```python
from build123d import *

# Parameters (mm, degrees)
M6X0P35_MALE_THREAD_MAJOR_ENVELOPE_START = 0.8
SKETCH1_R                                = 3
SKETCH1_R_2                              = 2.2
M6X0P35_MALE_THREAD_MAJOR_ENVELOPE_DEPTH = 1.4
BALL_RETENTION_CAP_FLANGE_START          = 2.2
SKETCH2_R                                = 3.5
SKETCH2_R_2                              = 2.2
BALL_RETENTION_CAP_FLANGE_DEPTH          = 0.5
SKETCH3_W                                = 0.45
SKETCH3_H                                = 0.6
OPPOSED_PIN_TOOL_NOTCHES_DEPTH           = 0.5


# Read off the part's stored shape, not the designer's step: Upper_Spherical_Bearing_Seat_D5p05
with BuildPart() as part:
    # Sketch1 → M6x0p35_Male_Thread_Major_Envelope (new body)
    with BuildSketch(Plane.XY.offset(M6X0P35_MALE_THREAD_MAJOR_ENVELOPE_START)):
        Circle(SKETCH1_R)
        Circle(SKETCH1_R_2, mode=Mode.SUBTRACT)
    extrude(amount=M6X0P35_MALE_THREAD_MAJOR_ENVELOPE_DEPTH)

    # Sketch2 → Ball_Retention_Cap_Flange (add)
    with BuildSketch(Plane.XY.offset(BALL_RETENTION_CAP_FLANGE_START)):
        Circle(SKETCH2_R)
        Circle(SKETCH2_R_2, mode=Mode.SUBTRACT)
    extrude(amount=BALL_RETENTION_CAP_FLANGE_DEPTH)

    # Upper_Spherical_Bearing_Seat_D5p05 outli → Upper_Spherical_Bearing_Seat_D5p05 (revolve, cut)
    with BuildSketch(Plane.XZ):
        with BuildLine():
            Line((2.199999999, 0.799999998), (2.394916492, 0.799999998))
            ThreePointArc((2.394916492, 0.799999998), (2.307929655, 1.024248851), (2.199999999, 1.239203375))
            Line((2.199999999, 1.239203375), (2.199999999, 0.799999998))
        make_face()
    revolve(axis=Axis((0, 0, 0), (0, 0, 1)), mode=Mode.SUBTRACT)

    # Sketch3 → Opposed_Pin_Tool_Notches (cut)
    with BuildSketch(Plane.XY.offset(2.7)):
        with Locations((-3.375, 0)):
            Rectangle(SKETCH3_W, SKETCH3_H)
        with Locations((3.375, 0)):
            Rectangle(SKETCH3_W, SKETCH3_H)
    extrude(amount=-OPPOSED_PIN_TOOL_NOTCHES_DEPTH, mode=Mode.SUBTRACT)


solid = part.part
```
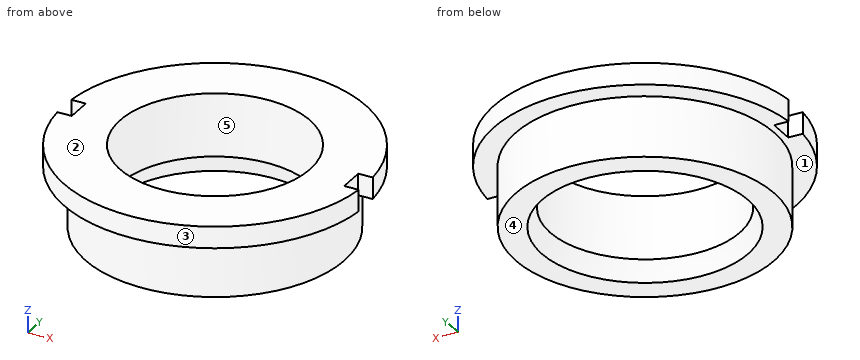
The model under review builds one solid part; all positions refer to its coordinate system, in mm. Face numbers are marked on the shaded views. A direction names the side the tool comes from. Round coordinates to 2 decimals unless told otherwise and drop trailing zeros. Loops run counter-clockwise (first coordinate to the right, second up) from the corner with the lowest first, then second, coordinate; pieces in that order, holes last. Notation, with made-up numbers: (87, -25.75) - (113, -25.75) arc R22 ccw to (113, 2.25) - close; hole circle Ø8 at (65.5, 41.5). An arc over 180 degrees is marked (long way). Write each question's results on one line, items separated by ' | '. Start each with the question number.
Q1. Take a section at D-D on y = -2.5. Give the boundary of the cut face in (x, z), plus the area to 3 significant figures.
Q2. Wall thickness on line 1 along Y through (x, z) = (0, 1.55); line 2 along X through (y, z) = (0.5, 1.2); line 3 along Y through (x, z) = (-1.75, 1.35): over which ranges is each line inside the solid? List them lowest first. Write a range as [from, to].
Q3. Take a section at C-C on x = 0.75. Give the boundary of the cut face in (y, z), plus the area to 3 significant figures.
Q4. Tool access review of the marked faces 1 and 2: name each direction out of +Z, -Z, +X, -X, +Y, -Y from which nothing blocks a thin tool from reaching the whole face with its end or side.
Q5. Take a section at B-B on y = 0. Give the boundary of the cut face in (x, z) (3 decimals).
Q6. Draft analysis for pull direction Y (two halves, no side actions). For the marked faces 3, 4 and 5, state which applies: pulls with the +Y half, pulls with the -Y half, needs draft (parallel to the pull), parting line crosses it, or undercut.
Data:
1) outline: (-2.45, 2.2) - (-1.66, 2.2) - (-1.66, 0.8) - (1.66, 0.8) - (1.66, 2.2) - (2.45, 2.2) - (2.45, 2.7) - (-2.45, 2.7) - close | area: 7.09 mm²
2) line 1: y = [-3, -2.2], [2.2, 3] | line 2: x = [-2.96, -2.16], [2.16, 2.96] | line 3: y = [-2.44, -1.33], [1.33, 2.44]
3) outline: (-3.42, 2.2) - (-2.9, 2.2) - (-2.9, 0.8) - (-2.27, 0.8) arc R2.41 cw to (-2.07, 1.24) - (-2.07, 2.7) - (-3.42, 2.7) - close; (2.07, 1.24) arc R2.41 cw to (2.27, 0.8) - (2.9, 0.8) - (2.9, 2.2) - (3.42, 2.2) - (3.42, 2.7) - (2.07, 2.7) - close | area: 3.59 mm²
4) face 1: -Z | face 2: +Z, +X, -X, +Y, -Y
5) outline: (-3.15, 2.2) - (-3, 2.2) - (-3, 0.8) - (-2.395, 0.8) arc R2.525 cw to (-2.2, 1.239) - (-2.2, 2.7) - (-3.15, 2.7) - close; (2.2, 1.239) arc R2.525 cw to (2.395, 0.8) - (3, 0.8) - (3, 2.2) - (3.15, 2.2) - (3.15, 2.7) - (2.2, 2.7) - close
6) face 3: pulls with the -Y half | face 4: needs draft | face 5: undercut
